Can you work these out from the model? Positions are in its coordinate system, mm. A direction names the side the tool comes from. Round coordinates to 2 decimals unless told otherwise and drop trailing zeros. Loops run counter-clockwise (first coordinate to the right, second up) from the corner with the lowest first, then second, coordinate; pieces in that order, holes last.
Autodesk Inventor part; units mm, degrees
ref_plane "YZ Plane" through (0, 0, 0) normal (1, 0, 0) x (0, 1, 0)
ref_plane "XZ Plane" through (0, 0, 0) normal (0, 1, 0) x (-1, 0, 0)
ref_plane "XY Plane" through (0, 0, 0) normal (0, 0, 1) x (1, 0, 0)
sketch "Náčrt2" plane through (0, 0, 0) normal (0, 0, 1) x (1, 0, 0)
  arc A0 (30, 0) -> (-30, 0) centre (0, 0) ccw
  arc A1 (40, 0) -> (-40, 0) centre (0, 0) ccw
  line L0 (-40, 0) -> (-30, 0)
  line L1 (30, 0) -> (40, 0)
  point P0 (-40, 0)
  dimension "d0" = 30
  dimension "d1" = 40
  dimension "d2" = 0
  dimension "d3" = 0
  dimension "d4" = 0
  dimension "d5" = 0
  dimension "d6" = 30
  dimension "d7" = 40
extrude "Vysunutí1" add sketch "Náčrt2" against normal blind 60
sketch "Náčrt3" plane through (30, 0, 0) normal (0, -1, 0) x (1, 0, 0)
  line L0 (10, 0) -> (-70, 0)
  line L1 (0, 0) -> (0, -60)
  line L2 (0, -60) -> (10, -60)
  line L3 (0, 0) -> (10, 0)
  line L4 (10, 0) -> (10, -60)
  line L5 (10, -60) -> (10, -60)
  line L6 (20, -50) -> (30, -50)
  line L7 (30, -10) -> (20, -10)
  line L8 (10, 0) -> (10, 0)
  arc A0 (30, -50) -> (30, -10) centre (30, -30) ccw
  circle A1 centre (30, -30) radius 8
  arc A2 (20, -50) -> (10, -60) centre (20, -60) ccw
  arc A3 (10, 0) -> (20, -10) centre (20, 0) ccw
  line L9 (-30, 0) -> (-30, -60)
  line L10 (-60, 0) -> (-60, -60)
  line L11 (-60, -60) -> (-70, -60)
  line L12 (-60, 0) -> (-70, 0)
  line L13 (-70, 0) -> (-70, -60)
  line L14 (-70, -60) -> (-70, -60)
  line L15 (-80, -50) -> (-90, -50)
  line L16 (-90, -10) -> (-80, -10)
  line L17 (-70, 0) -> (-70, 0)
  arc A4 (-90, -10) -> (-90, -50) centre (-90, -30) ccw
  circle A5 centre (-90, -30) radius 8
  arc A6 (-70, -60) -> (-80, -50) centre (-80, -60) ccw
  arc A7 (-80, -10) -> (-70, 0) centre (-80, 0) ccw
  point P0 (10, -50)
  point P1 (10, -10)
  point P2 (-70, -50)
  point P3 (-70, -10)
  dimension "d10" = 10
  dimension "d12" = 16
  dimension "d13" = 10
  dimension "d16" = 20
  dimension "d17" = 30
extrude "Vysunutí2" add sketch "Náčrt3" against normal blind 10
sketch "Sketch4" plane through (0, 0, -60) normal (0, 0, -1) x (-1, 0, 0)
  arc A0 (38.7298, 10) -> (-38.7298, 10) centre (0, 0) ccw
  line L0 (-38.7298, 10) -> (-25, 100)
  line L1 (25, 100) -> (38.7298, 10)
  arc A1 (38.7298, 10) -> (-38.7298, 10) centre (0, -0.1304) ccw
  line L2 (30, 0) -> (40, 0)
  arc A2 (-25, 100) -> (25, 100) centre (0, 100) ccw
  arc A3 (-15, 100) -> (15, 100) centre (0, 100) ccw
  line L3 (-25, 100) -> (-15, 100)
  line L4 (15, 100) -> (25, 100)
  line L5 (-5, 75.5051) -> (5, 75.5051)
  line L6 (-5, 75.5051) -> (-5, 39.589)
  line L7 (5, 75.5051) -> (5, 39.589)
  line L8 (-5, 39.589) -> (5, 39.589)
  point P0 (5, 39.6863)
  point P1 (-5, 39.6863)
  dimension "d20" = 50
  dimension "d24" = 15
  dimension "d36" = 100
  dimension "d37" = 30
  dimension "d48" = 10
  dimension "d49" = 40.0328
  dimension "d50" = 39.6863
  dimension "d51" = 39.6863
  dimension "d52" = 28.8671
  dimension "d53" = 38.7527
extrude "Extrusion3" add sketch "Sketch4" against normal blind 10 contours A0 L7 A2 L1 | A0 L0 A2 L6
extrude "Extrusion4" add sketch "Sketch4" against normal blind 30 contours A2 L5 L3 A3 L4
extrude "Extrusion5" add sketch "Sketch4" against normal blind 60 contours L7 A1 L6 A0 | A0 L6 A2 L7 | L8 A1 | A2 L5
sketch "Sketch5" plane through (5, 39.6863, -50) normal (1, 0, 0) x (0, 0, -1)
  line L0 (-50, 0) -> (-50, 35.8188)
  line L1 (0, 35.8188) -> (-20, 35.8188)
  line L2 (-50, 0) -> (-20, 35.8188)
  line L3 (-20, 35.8188) -> (-50, 35.8188)
  line L4 (-50, 35.8188) -> (-50, 0)
  point P0 (-50, -39.6863)
extrude "Extrusion6" cut sketch "Sketch5" against normal blind 10
properties part number "4"
(1) If we mould it in two halves opening along X, with no side actions, what happens to faces 1 (the cylindrical face through (80, 5, -30)), 2 (the flat face through (0.07, 57.345, -14.79)), 3 (the cylindrical face through (0.66, 29.993, -29.58))? For each: released by +X, released by -X, zero draft, split by the parting line, or undercut.
Worked answers:
face 1: released by +X
face 2: zero draft
face 3: undercut
(2) If we section it at D-D, the plane y = 37: List the corners of the cut face in (x, z) for me.
Worked answers:
outline: (-34.61, -60) - (34.61, -60) - (34.61, -50) - (15.2, -50) - (15.2, 0) - (-15.2, 0) - (-15.2, -50) - (-34.61, -50) - close
(3) Will these pins go through, and if not, where does the flat tip stop? P1, Ø17, axis at x = -16.5, y = 65, coming from the +Z side; P2, Ø18, axis at y = 62.5, z = -17, coming from the -X side; P3, Ø19.5, axis at x = 2.5, y = 84, coming from the +Z side; P4, Ø18.5, axis at x = -60, z = -30, coming from the -Y side.
Worked answers:
P1: stops at z = -50
P2: stops at x = -5
P3: stops at z = -28.95
P4: stops at y = 0
(4) For faces 4 (the cylindrical face through (19.516, 84.375, -40.14)), 5 (the flat face through (-55, 5, -50)), 6 (the cylindrical face through (-26.176, 30.246, -29.58)), 7 (the flat face through (-55, 5, -10)), which set-ups out of +Z, -Z, +X, -X, +Y, -Y let a thin tool reach every point of the face, with its end or its side?
Worked answers:
face 4: +Z, +X
face 5: -Z, -X, +Y, -Y
face 6: +Z, -X
face 7: +Z, -X, +Y, -Y
(5) If we section it at B-B, the plane x = 0: List the corners of the cut face in (y, z) for me, then the cut area to 3 significant figures.
Worked answers:
outline: (30, -60) - (85, -60) - (85, -30) - (75.51, -30) - (39.69, 0) - (30, 0) - close
area: 2,480 mm2
(6) If we section it at A-A, the plane y = 21: List the corners of the cut face in (x, z) for me.
Worked answers:
outline: (-37.05, -60) - (-21.42, -60) - (-21.42, 0) - (-34.04, 0) - (-34.04, -50) - (-37.05, -50) - close; (21.42, -60) - (37.05, -60) - (37.05, -50) - (34.04, -50) - (34.04, 0) - (21.42, 0) - close
(7) If I drill on line 1 (Z direction, x = -60, y = 3.25); line 2 (Z direction, x = -50, y = 5); line 3 (Y direction, x = 51.5, z = -20), over which ranges is the centre line in solid material (lowest first)?
Worked answers:
line 1: z = -50 to -38, -22 to -10
line 2: z = -50 to -10
line 3: y = 0 to 10
(8) If we section it at C-C, the plane x = 58: List the corners of the cut face in (y, z) for me.
Worked answers:
outline: (0, -50) - (10, -50) - (10, -37.75) - (0, -37.75) - close; (0, -22.25) - (10, -22.25) - (10, -10) - (0, -10) - close
